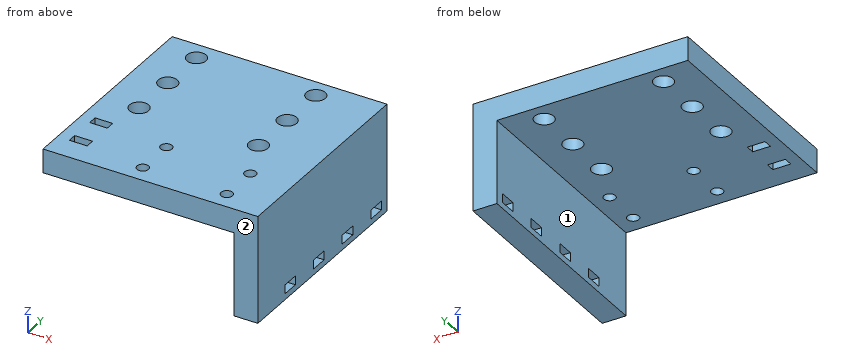
from build123d import *

# Parameters (mm, degrees)
SKETCH1_W           = 50.8
SKETCH1_H           = 57.15
BOSS_EXTRUDE1_DEPTH = 6.35
SKETCH5_R           = 1.524
SKETCH5_R_2         = 2.54
CUT_EXTRUDE1_DEPTH  = 72.447438113
SKETCH6_W           = 4.7625
SKETCH6_H           = 2.38125
SKETCH6_W_2         = 4.700923451
CUT_EXTRUDE2_DEPTH  = 72.447438113
SKETCH9_W           = 28.575
SKETCH9_H           = 57.15
BOSS_EXTRUDE2_DEPTH = 6.35
SKETCH11_W          = 2.38252
SKETCH11_H          = 4.70154
CUT_EXTRUDE4_DEPTH  = 75.015666563
LPATTERN1_COUNT     = 4
LPATTERN1_PITCH     = 12.7


with BuildPart() as part:
    # Sketch1 → Boss-Extrude1 (new body)
    with BuildSketch(Plane.XY):
        with Locations((-32.446072824, -12.876728212)):
            Rectangle(SKETCH1_W, SKETCH1_H)
    extrude(amount=BOSS_EXTRUDE1_DEPTH)

    # Sketch5 → Cut-Extrude1 (cut, through all)
    with BuildSketch(Plane.XY.offset(6.35)):
        with Locations((-11.808572824, -26.275228212)):
            Circle(SKETCH5_R)
        with Locations((-11.808572824, -36.689228212)):
            Circle(SKETCH5_R)
        with Locations((-34.160572824, -26.275228212)):
            Circle(SKETCH5_R)
        with Locations((-34.160572824, -36.689228212)):
            Circle(SKETCH5_R)
        with Locations((-48.321072824, 10.618271788)):
            Circle(SKETCH5_R_2)
        with Locations((-16.571072824, 10.618271788)):
            Circle(SKETCH5_R_2)
        with Locations((-48.321072824, -2.081728212)):
            Circle(SKETCH5_R_2)
        with Locations((-16.571072824, -2.081728212)):
            Circle(SKETCH5_R_2)
        with Locations((-48.321072824, -14.781728212)):
            Circle(SKETCH5_R_2)
        with Locations((-16.571072824, -14.781728212)):
            Circle(SKETCH5_R_2)
    extrude(amount=-CUT_EXTRUDE1_DEPTH, mode=Mode.SUBTRACT)

    # Sketch6 → Cut-Extrude2 (cut, through all)
    with BuildSketch(Plane.XY.offset(6.35)):
        with Locations((-52.289822824, -33.911103212)):
            Rectangle(SKETCH6_W, SKETCH6_H)
        with Locations((-52.320611099, -24.900183987)):
            Rectangle(SKETCH6_W_2, SKETCH6_H)
    extrude(amount=-CUT_EXTRUDE2_DEPTH, mode=Mode.SUBTRACT)

    # Sketch9 → Boss-Extrude2 (add)
    with BuildSketch(Plane(origin=(-7.046072824, 0, 0), x_dir=(0, 0, -1), z_dir=(1, 0, 0))):
        with Locations((7.9375, -12.876728212)):
            Rectangle(SKETCH9_W, SKETCH9_H)
    extrude(amount=BOSS_EXTRUDE2_DEPTH)

    # Sketch11 → Cut-Extrude4 (cut, through all)
    with BuildSketch(Plane(origin=(-0.696072824, 0, 0), x_dir=(0, 0, -1), z_dir=(1, 0, 0))):
        with Locations((19.44624, 10.915505986)):
            Rectangle(SKETCH11_W, SKETCH11_H)
    cut_extrude4 = extrude(amount=-CUT_EXTRUDE4_DEPTH, mode=Mode.SUBTRACT)

    # LPattern1: Cut-Extrude4 ×4
    with Locations(*[(0, -i * LPATTERN1_PITCH, 0) for i in range(1, LPATTERN1_COUNT)]):
        add(cut_extrude4, mode=Mode.SUBTRACT)


solid = part.part
Read the model definition and answer for the solid it produces. Units are mm, in the model's axes. Face numbers are marked on the shaded views. A direction names the side the tool comes from. Give positions to 0.01 mm unless a question says otherwise; leave off trailing zeros. Write each loop counter-clockwise with the first axis right and the second up, starting at its lowest first coordinate (ties: lowest second). Pieces come first, ordered by that corner, then holes. Notation, with made-up numbers: (-23.75, 58) - (9.25, 58) arc R8 cw to (9.25, 71) - close; hole circle Ø4 at (60, 60.5). An arc over 180 degrees is marked (long way). Use CSV: the item, a comma, the result in double quotes. Start each with the question number.
(1) Find section D-D (z = -11.75). Give the vertices of the cut face in (x, y).
(2) For the marked faces 1 and 2, determine the directions among +Z, -Z, +X, -X, +Y, -Y from which every point of the face is accessible in a straight line to the end or side of a thin tool.
(3) Given P1, Ø1.5, axis at x = -19.5, y = -27, coming from the -Z side; P2, Ø6.5, axis at y = -10.5, z = -14.5, coming from the -X side; P3, Ø4.5, axis at x = -48.32, y = -2.08, coming from the +Z side, each flat-ended and moving along its own axis, determine where each tip first touches the part or whether it passes through.
(4) Find section A-A (x = -12.5). Give the vertices of the cut face in (y, z), plus the area to 3 significant figures.
(5) Find section B-B (y = -21.5). Give the vertices of the cut face in (x, z) (3 decimals), plus the area to 3 significant figures.
(6) Consider line 1 along Y through (x, z) = (-16.5, 5); line 2 along X through (y, z) = (-30, -19.75); line 3 along Z through (x, y) = (-36, 3.5). Determine where each line is inside the solid, lowest interval first.
(7) Find section C-C (y = -37.5). Give the vertices of the cut face in (x, z) (3 decimals).
Findings below:
1,outline,"(-7.05, -41.45) - (-0.7, -41.45) - (-0.7, 15.7) - (-7.05, 15.7) - close"
2,face 1,"-Z, -X, +Y, -Y"
2,face 2,"+Z, -Z, +X, -X, -Y"
3,P1,"z = 0"
3,P2,"x = -7.05"
3,P3,"through"
4,outline,"(-41.45, 0) - (-38.05, 0) - (-38.05, 6.35) - (-41.45, 6.35) - close; (-35.33, 0) - (-27.63, 0) - (-27.63, 6.35) - (-35.33, 6.35) - close; (-24.92, 0) - (15.7, 0) - (15.7, 6.35) - (-24.92, 6.35) - close"
4,area,"328 mm2"
5,outline,"(-57.846, 0) - (-7.046, 0) - (-7.046, -22.225) - (-0.696, -22.225) - (-0.696, 6.35) - (-57.846, 6.35) - close"
5,area,"504 mm2"
6,line 1,"-41.45 to -17.32, -12.24 to -4.62, 0.46 to 8.08, 13.16 to 15.7"
6,line 2,"-7.05 to -0.7"
6,line 3,"0 to 6.35"
7,outline,"(-57.846, 0) - (-35.451, 0) - (-35.451, 6.35) - (-57.846, 6.35) - close; (-32.87, 0) - (-13.099, 0) - (-13.099, 6.35) - (-32.87, 6.35) - close; (-10.518, 0) - (-7.046, 0) - (-7.046, -22.225) - (-0.696, -22.225) - (-0.696, 6.35) - (-10.518, 6.35) - close"
